Here's how the part is built. I have some questions about the finished solid (model axes, mm). A direction names the side the tool comes from. Give positions to 0.01 mm unless a question says otherwise; leave off trailing zeros. Write each loop counter-clockwise with the first axis right and the second up, starting at its lowest first coordinate (ties: lowest second). Pieces come first, ordered by that corner, then holes. Notation, with made-up numbers: (-19.5, 58) -> (29.5, 58) arc R31 ccw to (29.5, 92) -> close; hole circle Ø4 at (59, 40.5). An arc over 180 degrees is marked (long way). Use one line per item in the form item = value.
```python
from build123d import *

# Parameters (mm, degrees)
BOSS_EXTRUDE1_DEPTH = 16
CUT_EXTRUDE2_REACH  = 149.03
SKETCH5_R           = 1.25
SKETCH5_W           = 12.5
SKETCH5_H           = 31
SKETCH5_3_R         = 1.5
CUT_EXTRUDE3_DEPTH  = 148.030473032
CUT_EXTRUDE1_REACH  = 99.211
SKETCH3_R           = 1.25


with BuildPart() as part:
    # Sketch1 → Boss-Extrude1 (new, symmetric)
    with BuildSketch(Plane.XY):
        Polygon((-56, 0), (-56, 60), (67.4, 60), (67.4, 0), (71.4, 0), (71.4, 64), (-60, 64), (-60, 0), align=None)
    extrude(amount=BOSS_EXTRUDE1_DEPTH, both=True)

    # Sketch5 → Cut-Extrude2 (cut, up to next)
    with BuildSketch(Plane(origin=(71.4, 0, 0), x_dir=(0, 0, -1), z_dir=(1, 0, 0)), mode=Mode.PRIVATE) as cut_extrude2_sk1:
        with Locations(Location((0, 1.875, 0), (0, 0, 90))):
            Circle(SKETCH5_R)
    cut_extrude2_tool1 = extrude(cut_extrude2_sk1.sketch, amount=-CUT_EXTRUDE2_REACH, mode=Mode.PRIVATE) & part.part
    # Sketch5 → Cut-Extrude2 (cut, up to next)
    with BuildSketch(Plane(origin=(71.4, 0, 0), x_dir=(0, 0, -1), z_dir=(1, 0, 0)), mode=Mode.PRIVATE) as cut_extrude2_sk2:
        with Locations((0, 38.125)):
            Circle(SKETCH5_R)
    cut_extrude2_tool2 = extrude(cut_extrude2_sk2.sketch, amount=-CUT_EXTRUDE2_REACH, mode=Mode.PRIVATE) & part.part
    # Sketch5 → Cut-Extrude2 (cut, up to next)
    with BuildSketch(Plane(origin=(71.4, 0, 0), x_dir=(0, 0, -1), z_dir=(1, 0, 0)), mode=Mode.PRIVATE) as cut_extrude2_sk3:
        with Locations((0, 20)):
            Rectangle(SKETCH5_W, SKETCH5_H)
    cut_extrude2_tool3 = extrude(cut_extrude2_sk3.sketch, amount=-CUT_EXTRUDE2_REACH, mode=Mode.PRIVATE) & part.part
    add(cut_extrude2_tool1.solids().sort_by_distance((71.4, 1.875, 0))[0], mode=Mode.SUBTRACT)
    add(cut_extrude2_tool2.solids().sort_by_distance((71.4, 38.125, 0))[0], mode=Mode.SUBTRACT)
    add(cut_extrude2_tool3.solids().sort_by_distance((71.4, 20, 0))[0], mode=Mode.SUBTRACT)

    # Sketch5_3 → Cut-Extrude3 (cut, through all)
    with BuildSketch(Plane(origin=(71.4, 0, 0), x_dir=(0, 0, -1), z_dir=(1, 0, 0))):
        with Locations(Location((0, 15.075, 0), (0, 0, 90))):
            Circle(SKETCH5_3_R)
    extrude(amount=-CUT_EXTRUDE3_DEPTH, mode=Mode.SUBTRACT)

    # Sketch3 → Cut-Extrude1 (cut, up to next)
    with BuildSketch(Plane(origin=(0, 64, 0), x_dir=(1, 0, 0), z_dir=(0, 1, 0)), mode=Mode.PRIVATE) as cut_extrude1_sk1:
        with Locations(Location((-12.070312755, 12.070312755, 0), (0, 0, 270))):
            Circle(SKETCH3_R)
    cut_extrude1_tool1 = extrude(cut_extrude1_sk1.sketch, amount=-CUT_EXTRUDE1_REACH, mode=Mode.PRIVATE) & part.part
    # Sketch3 → Cut-Extrude1 (cut, up to next)
    with BuildSketch(Plane(origin=(0, 64, 0), x_dir=(1, 0, 0), z_dir=(0, 1, 0)), mode=Mode.PRIVATE) as cut_extrude1_sk2:
        with Locations(Location((12.070312755, 12.070312755, 0), (0, 0, 270))):
            Circle(SKETCH3_R)
    cut_extrude1_tool2 = extrude(cut_extrude1_sk2.sketch, amount=-CUT_EXTRUDE1_REACH, mode=Mode.PRIVATE) & part.part
    # Sketch3 → Cut-Extrude1 (cut, up to next)
    with BuildSketch(Plane(origin=(0, 64, 0), x_dir=(1, 0, 0), z_dir=(0, 1, 0)), mode=Mode.PRIVATE) as cut_extrude1_sk3:
        with Locations(Location((12.070312755, -12.070312755, 0), (0, 0, 270))):
            Circle(SKETCH3_R)
    cut_extrude1_tool3 = extrude(cut_extrude1_sk3.sketch, amount=-CUT_EXTRUDE1_REACH, mode=Mode.PRIVATE) & part.part
    # Sketch3 → Cut-Extrude1 (cut, up to next)
    with BuildSketch(Plane(origin=(0, 64, 0), x_dir=(1, 0, 0), z_dir=(0, 1, 0)), mode=Mode.PRIVATE) as cut_extrude1_sk4:
        with Locations(Location((-12.070312755, -12.070312755, 0), (0, 0, 270))):
            Circle(SKETCH3_R)
    cut_extrude1_tool4 = extrude(cut_extrude1_sk4.sketch, amount=-CUT_EXTRUDE1_REACH, mode=Mode.PRIVATE) & part.part
    # Sketch3 → Cut-Extrude1 (cut, up to next)
    with BuildSketch(Plane(origin=(0, 64, 0), x_dir=(1, 0, 0), z_dir=(0, 1, 0)), mode=Mode.PRIVATE) as cut_extrude1_sk5:
        Polygon((4.041451884, -7), (8.082903769, 0), (4.041451884, 7), (-4.041451884, 7), (-8.082903769, 0), (-4.041451884, -7), align=None)
    cut_extrude1_tool5 = extrude(cut_extrude1_sk5.sketch, amount=-CUT_EXTRUDE1_REACH, mode=Mode.PRIVATE) & part.part
    add(cut_extrude1_tool1.solids().sort_by_distance((-12.070313, 64, -12.070313))[0], mode=Mode.SUBTRACT)
    add(cut_extrude1_tool2.solids().sort_by_distance((12.070313, 64, -12.070313))[0], mode=Mode.SUBTRACT)
    add(cut_extrude1_tool3.solids().sort_by_distance((12.070313, 64, 12.070313))[0], mode=Mode.SUBTRACT)
    add(cut_extrude1_tool4.solids().sort_by_distance((-12.070313, 64, 12.070313))[0], mode=Mode.SUBTRACT)
    add(cut_extrude1_tool5.solids().sort_by_distance((0, 64, 0))[0], mode=Mode.SUBTRACT)


solid = part.part
```
Q1. I want a section at C-C, the plane z = -4. Write out the boundary of the cut face in (x, y), and give its area (3 significant figures).
Result set:
outline = (-60, 0) -> (-56, 0) -> (-56, 60) -> (-5.77, 60) -> (-5.77, 64) -> (-60, 64) -> close; (5.77, 60) -> (67.4, 60) -> (67.4, 35.5) -> (71.4, 35.5) -> (71.4, 64) -> (5.77, 64) -> close; (67.4, 0) -> (71.4, 0) -> (71.4, 4.5) -> (67.4, 4.5) -> close
area = 835 mm2
Q2. Which directions (+Z, -Z, +X, -X, +Y, -Y) give clear straight access to the entire face, cutting with the end or side of a thin tool? Please do faces 5 (the face through (67.4, 37, 4)), 6 (the face through (0, 62, 7)), 7 (the face through (69, 20, -6.25)), 8 (the face through (69, 0, 0)).
Result set:
face_5 = +Z, -Z, -Y
face_6 = +Y, -Y
face_7 = +X
face_8 = +Z, -Z, +X, -X, -Y
Q3. Will this pin go through, and if not, where does the flat tip stop? pin 1 Ø5 at (x, z) = (39.5, -3) entering from -Y.
Result set:
pin_1 = 60
Q4. If I drill on line 1 along X through (y, z) = (18.5, 10.5); line 2 along Y through (x, z) = (40.5, -3.5); line 3 along X through (y, z) = (7, -3), over which ranges is the centre line in solid material (lowest first)? Write a range as from..to.
Result set:
line_1 = -60..-56, 67.4..71.4
line_2 = 60..64
line_3 = -60..-56
Q5. I want a section at A-A, the plane y = 48.5. Write out the boundary of the cut face in (x, z).
Result set:
outline = (-60, -16) -> (-56, -16) -> (-56, 16) -> (-60, 16) -> close; (67.4, -16) -> (71.4, -16) -> (71.4, 16) -> (67.4, 16) -> close
Q6. I want a section at D-D, the plane x = 62.5. Write out the boundary of the cut face in (y, z).
Result set:
outline = (60, -16) -> (64, -16) -> (64, 16) -> (60, 16) -> close
Q7. If we mould it in two halves opening along Z, with no side actions, what happens to faces 1 (the face through (10.961, 62.028, 12.647)), 2 (the face through (-56, 30, 0)), 3 (the face through (1, 61, -16)), 4 (the face through (6.034, 62.028, 3.549))? For each: +Z half, -Z half, draft (parallel to the pull), parting line (faces both ways), or undercut.
Result set:
face_1 = undercut
face_2 = draft
face_3 = -Z half
face_4 = undercut
Q8. I want a section at B-B, the plane z = 8.5. Write out the boundary of the cut face in (x, y).
Result set:
outline = (-60, 0) -> (-56, 0) -> (-56, 60) -> (67.4, 60) -> (67.4, 0) -> (71.4, 0) -> (71.4, 64) -> (-60, 64) -> close
